from build123d import *

# Parameters (mm, degrees)
BOSS_EXTRUDE1_DEPTH  = 3
M6_CLEARANCE_HOLE1_D = 6.6
M6_CLEARANCE_HOLE2_D = 6.6
SKETCH6_R            = 3.75
CUT_EXTRUDE1_DEPTH   = 532.991776252
FILLET1_R            = 1


with BuildPart() as part:
    # Sketch1 → Boss-Extrude1 (new body)
    with BuildSketch(Plane.XY):
        Polygon((25.5, 522.5), (25.5, -25.5), (74.5, -25.5), (74.5, 0), (100, 0), (100, 497), (74.5, 497), (74.5, 522.5), align=None)
    extrude(amount=BOSS_EXTRUDE1_DEPTH)

    # M6 Clearance Hole1 (through all)
    with Locations(Plane(origin=(0, 0, 0), x_dir=(-1, 0, 0), z_dir=(0, 0, -1))):
        with Locations((-87.5, 12.5), (-87.5, 484.5), (-87.5, 248.5)):
            Hole(M6_CLEARANCE_HOLE1_D / 2)

    # M6 Clearance Hole2 (through all)
    with Locations(Plane(origin=(0, 0, 0), x_dir=(-1, 0, 0), z_dir=(0, 0, -1))):
        with Locations((-40.5, 248.5)):
            Hole(M6_CLEARANCE_HOLE2_D / 2)

    # Sketch6 → Cut-Extrude1 (cut, through all)
    with BuildSketch(Plane(origin=(0, 0, 0), x_dir=(-1, 0, 0), z_dir=(0, 0, -1))):
        with Locations((-25.5, -14)):
            Circle(SKETCH6_R)
        with Locations((-25.5, 511)):
            Circle(SKETCH6_R)
    extrude(amount=-CUT_EXTRUDE1_DEPTH, mode=Mode.SUBTRACT)

    # Fillet1
    fillet1_edges = [part.edges().sort_by_distance(p)[0] for p in [
        (74.5, -25.5, 1.5),
        (25.5, -25.5, 1.5),
        (25.5, 522.5, 1.5),
        (74.5, 522.5, 1.5),
        (74.5, 497, 1.5),
        (100, 497, 1.5),
        (100, 0, 1.5),
        (74.5, 0, 1.5),
        (25.5, -17.75, 1.5),
        (25.5, -10.25, 1.5),
        (25.5, 507.25, 1.5),
        (25.5, 514.75, 1.5),
    ]]
    fillet(fillet1_edges, radius=FILLET1_R)


solid = part.part
Geometry check sheet. Reference: the model listing, model coordinates, mm. Round coordinates to 2 decimals unless told otherwise and drop trailing zeros. Order: outer loops, then holes, each group sorted by start corner. A loop starts at its lowest first (then second) coordinate and runs counter-clockwise, first axis right, second up. Notation, with made-up numbers: M -17,79 L -9,79 A33 ccw -9,118 Z; hole C -11.75,-25.75 d9. An arc over 180 degrees is marked long. Answer in a Markdown table with one row per item. Add a question column.
Item 1: Material ranges on L1, parallel to Y at x = 87.5, z = 0.9; L2, parallel to X at y = 248.5, z = 1.65; L3, parallel to Y at x = 90.5, z = 2.2, recorded low to high. Write a range as [from, to].
Item 2: Depth check by flat-ended pin: pin 1 Ø5.5 at (x, y) = (87.5, 12.5) entering from +Z; pin 2 Ø0.9 at (x, z) = (87, 1.5) entering from -Y; pin 3 Ø1.5 at (y, z) = (-10.5, 2) entering from +X. Enter the tip coordinate at first touch or a pass-through.
Item 3: Sectioned sample at A-A, the plane z = 0.8. Enter the section's corners in (x, y).
Filled in:
| question | item | result |
|---|---|---|
| 1 | L1 | y = [0, 9.2], [15.8, 245.2], [251.8, 481.2], [487.8, 497] |
| 1 | L2 | x = [25.5, 37.2], [43.8, 84.2], [90.8, 100] |
| 1 | L3 | y = [0, 11.13], [13.87, 247.13], [249.87, 483.13], [485.87, 497] |
| 2 | pin 1 | passes through |
| 2 | pin 2 | stops at y = 0 |
| 2 | pin 3 | stops at x = 74.5 |
| 3 | outline | M 25.5,-24.5 A1 ccw 26.5,-25.5 L 73.5,-25.5 A1 ccw 74.5,-24.5 L 74.5,-1 A1 cw 75.5,0 L 99,0 A1 ccw 100,1 L 100,496 A1 ccw 99,497 L 75.5,497 A1 cw 74.5,498 L 74.5,521.5 A1 ccw 73.5,522.5 L 26.5,522.5 A1 ccw 25.5,521.5 L 25.5,515.64 A1 ccw 26.29,514.67 A3.75 cw 26.29,507.33 A1 ccw 25.5,506.36 L 25.5,-9.36 A1 ccw 26.29,-10.33 A3.75 cw 26.29,-17.67 A1 ccw 25.5,-18.64 Z; hole C 40.5,248.5 d6.6; hole C 87.5,12.5 d6.6; hole C 87.5,248.5 d6.6; hole C 87.5,484.5 d6.6 |
